For this review, use the dimensioned drawing (mm, ordinates from the lowest corner) and the shaded views. A direction names the side the tool comes from. Coordinates: 2 decimals unless noted, no trailing zeros. Write each loop counter-clockwise with the first axis right and the second up, starting at its lowest first coordinate (ties: lowest second). Pieces come first, ordered by that corner, then holes. Notation, with made-up numbers: (43.25, 21) - (50.25, 21) arc R15 ccw to (50.25, 36) - close; hole circle Ø2 at (51, -29). An arc over 180 degrees is marked (long way). Answer as a JSON object with one key per item and string values.
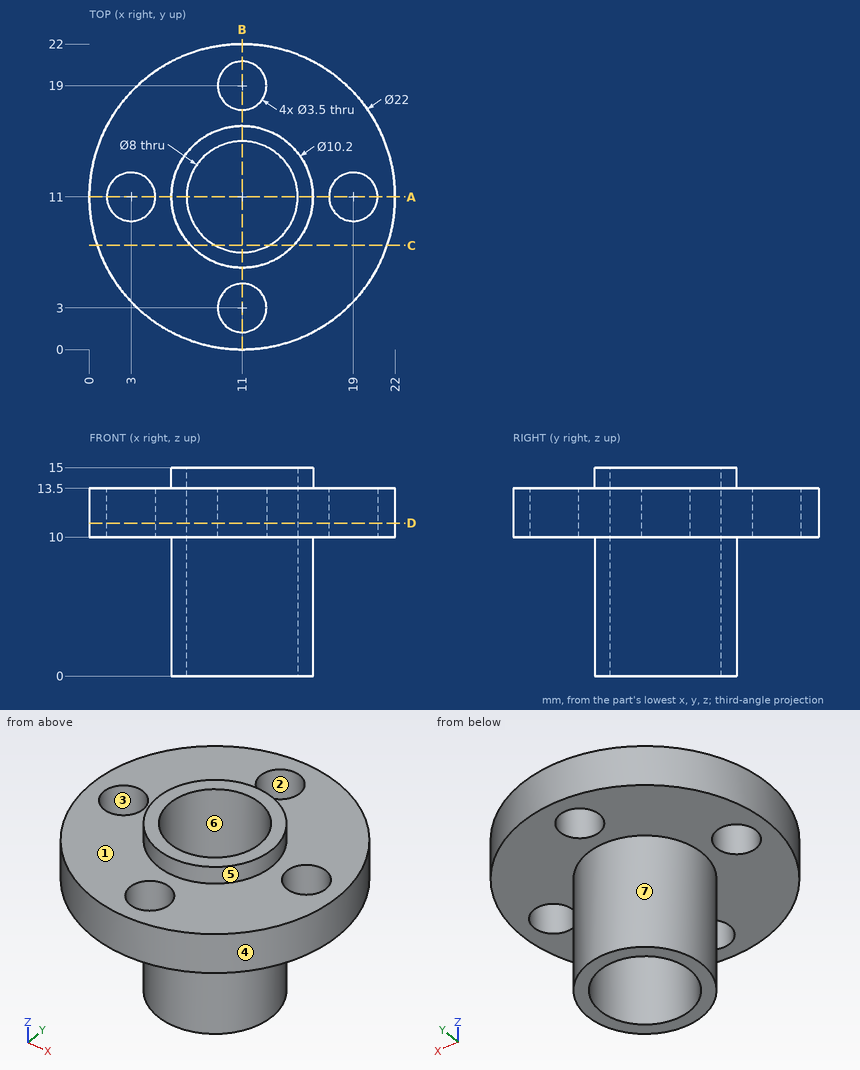
(1) For pin 1 (10 mm diameter, centred on x = 17.5, y = 18.5, fed in from +Z); pin 2 (8 mm diameter, centred on x = 14.5, z = 2.5, fed in from +Y); pin 3 (1 mm diameter, centred on x = 9.5, z = 13, fed in from +Y); pin 4 (5.5 mm diameter, centred on x = 11, y = 3, fed in from -Z), all flat-tipped, find the tip position at first contact; note any pin that passes through.
Solved:
{"pin 1": "stops at z = 15", "pin 2": "stops at y = 16.1", "pin 3": "stops at y = 21.95", "pin 4": "stops at z = 10"}
(2) Take a section at C-C, the plane y = 7.5. Write out the cut boundary in (x, z), and give its area (3 significant figures).
Solved:
{"outline": "(0.57, 10) - (7.29, 10) - (7.29, 0) - (9.06, 0) - (9.06, 15) - (7.29, 15) - (7.29, 13.5) - (0.57, 13.5) - close; (12.94, 0) - (14.71, 0) - (14.71, 10) - (21.43, 10) - (21.43, 13.5) - (14.71, 13.5) - (14.71, 15) - (12.94, 15) - close", "area": "100 mm^2"}
(3) Tool access review of the marked faces 5, 6 and 7: name each direction out of +Z, -Z, +X, -X, +Y, -Y from which nothing blocks a thin tool from reaching the whole face with its end or side.
Solved:
{"face 5": "+Z", "face 6": "+Z, -Z", "face 7": "-Z"}
(4) The part is to be moulded in two halves that separate along X. For the marked faces 1, 2, 3 and 4, say which applies: pulls with the +X half, pulls with the -X half, needs draft (parallel to the pull), parting line crosses it, or undercut.
Solved:
{"face 1": "needs draft", "face 2": "undercut", "face 3": "undercut", "face 4": "parting line crosses it"}
(5) Take a section at D-D, the plane z = 11. Write out the cut boundary in (x, y).
Solved:
{"outline": "circle Ø22 at (11, 11); hole circle Ø3.5 at (3, 11); hole circle Ø8 at (11, 11); hole circle Ø3.5 at (11, 3); hole circle Ø3.5 at (11, 19); hole circle Ø3.5 at (19, 11)"}
(6) Take a section at A-A, the plane y = 11. Write out the cut boundary in (x, z), and give its area (3 significant figures).
Solved:
{"outline": "(0, 10) - (1.25, 10) - (1.25, 13.5) - (0, 13.5) - close; (4.75, 10) - (5.9, 10) - (5.9, 0) - (7, 0) - (7, 15) - (5.9, 15) - (5.9, 13.5) - (4.75, 13.5) - close; (15, 0) - (16.1, 0) - (16.1, 10) - (17.25, 10) - (17.25, 13.5) - (16.1, 13.5) - (16.1, 15) - (15, 15) - close; (20.75, 10) - (22, 10) - (22, 13.5) - (20.75, 13.5) - close", "area": "49.8 mm^2"}
(7) To check wall thickness, follow line 1 (X direction, y = 10.5, z = 12.75); line 2 (Y direction, x = 12, z = 12.25); line 3 (Y direction, x = 11, z = 8). State the ranges of each line that lie inside material, in increasing order. Write a range as from..to.
Solved:
{"line 1": "x = 0.01..1.32, 4.68..7.03, 14.97..17.32, 20.68..21.99", "line 2": "y = 0.05..1.56, 4.44..7.13, 14.87..17.56, 20.44..21.95", "line 3": "y = 5.9..7, 15..16.1"}
